Read the model definition and answer for the solid it produces. Units are mm, in the model's axes. Round coordinates to 2 decimals unless told otherwise and drop trailing zeros. Loops run counter-clockwise (first coordinate to the right, second up) from the corner with the lowest first, then second, coordinate; pieces in that order, holes last. Notation, with made-up numbers: M 81,60.5 L 138,60.5 A26 cw 138,95.5 Z; hole C 82.25,64.5 d1. An arc over 180 degrees is marked long. Write each question's results on one line, items separated by ' | '.
```python
from build123d import *

# Parameters (mm, degrees)
F0_R     = 16.5
F1_DEPTH = 1060
F2_R     = 21
F3_DEPTH = 500
F5_DEPTH = 50


with BuildPart() as f1:
    # F0 (on Front) → F1 (new body)
    with BuildSketch(Plane.XZ):
        Circle(F0_R)
    extrude(amount=F1_DEPTH)

    # F2 (on Top) → F3 (cut, symmetric)
    with BuildSketch(Plane.XY):
        Circle(F2_R)
    extrude(amount=F3_DEPTH, both=True, mode=Mode.SUBTRACT)

    # F4 (on Top) → F5 (cut, symmetric)
    with BuildSketch(Plane.XY):
        with BuildLine():
            Line((-21, -1060), (0, -1060))
            Line((0, -1060), (21, -1060))
            ThreePointArc((21, -1060), (0, -1039), (-21, -1060))
        make_face()
    extrude(amount=F5_DEPTH, both=True, mode=Mode.SUBTRACT)


solid = f1.part
```
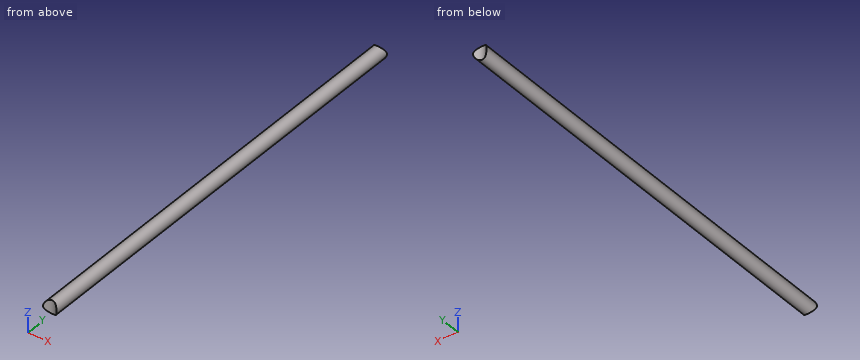
1. Find the intervals of material crossed by L1, parallel to X at y = -162, z = -2.5; L2, parallel to X at y = -73.5, z = -1; L3, parallel to Z at x = 5.5, y = -117, in increasing order.
Completed:
L1: x = -16.31 to 16.31 | L2: x = -16.47 to 16.47 | L3: z = -15.56 to 15.56
2. Find section C-C, the plane z = -7.5. Give the vertices of the cut face in (x, y), then the cut area to 3 significant figures.
Completed:
outline: M -14.7,-1045 A21 cw 14.7,-1045 L 14.7,-15 A21 cw -14.7,-15 Z | area: 30,000 mm2
3. Find section A-A, the plane y = -961.5. Give the vertices of the cut face in (x, z).
Completed:
outline: C 0,0 d33
4. Find section B-B, the plane x = 0. Give the vertices of the cut face in (y, z).
Completed:
outline: M -1039,-16.5 L -21,-16.5 L -21,16.5 L -1039,16.5 Z
5. Given P1, Ø2, axis at x = -5.5, y = -759.5, coming from the -Z side; P2, Ø4, axis at x = -7.5, z = -0.5, coming from the -Y side; P3, Ø1.5, axis at x = -4.5, y = -367.5, coming from the -Z side, each flat-ended and moving along its own axis, determine where each tip first touches the part or whether it passes through.
Completed:
P1: stops at z = -15.87 | P2: stops at y = -1041.27 | P3: stops at z = -16.07
